The listing builds one solid part. Answer for the finished solid, in the listing's coordinates (mm). Round coordinates to 2 decimals unless told otherwise and drop trailing zeros. Loops run counter-clockwise (first coordinate to the right, second up) from the corner with the lowest first, then second, coordinate; pieces in that order, holes last. Notation, with made-up numbers: (34, 25) - (52, 25) arc R26 cw to (52, 51) - close; hole circle Ø3 at (-26.5, 60). An arc over 180 degrees is marked (long way). One line per item, written item: value.
```python
from build123d import *

# Parameters (mm, degrees)
CYLINDER964_R          = 74
CYLINDER964_DEPTH      = 32
BOX476_W               = 50
BOX476_H               = 6
BOX476_DEPTH           = 26
CUT443_PLACEMENT_ANGLE = 90


with BuildPart() as obj1:
    # Cylinder964 → Cylinder964 (new body)
    with BuildSketch(Plane.XY.offset(50)):
        Circle(CYLINDER964_R)
    extrude(amount=CYLINDER964_DEPTH)


with BuildPart() as cut443:
    # Box476 → Box476 (new body)
    with BuildSketch(Plane(origin=(-112, -24, 56), x_dir=(1, 0, 0), z_dir=(0, 0, 1))):
        with Locations((25, 3)):
            Rectangle(BOX476_W, BOX476_H)
    extrude(amount=BOX476_DEPTH)

    # Cut443: cut obj1
    add(obj1.part, mode=Mode.SUBTRACT)


with BuildPart() as cut443_1:
    # Cut443 placement: moved
    add(cut443.part.rotate(Axis((0, 0, 0), (0, 0, 1)), CUT443_PLACEMENT_ANGLE))


solid = cut443_1.part
```
1) A cutting plane is placed at B-B on x = 21. Give the vertices of the cut face in (y, z), and give its area (3 significant figures).
Final values:
outline: (-112, 56) - (-70.96, 56) - (-70.96, 82) - (-112, 82) - close
area: 1,070 mm2
2) This flat-tipped pin is pushed along its axis until it touches: pin 1 Ø3 at (x, z) = (23, 75.5) entering from +Y. Where does it stop, or does it pass through?
Final values:
pin 1: y = -70
3) A cutting plane is placed at A-A on z = 59.5. Give the vertices of the cut face in (x, y), and give its area (3 significant figures).
Final values:
outline: (18, -112) - (24, -112) - (24, -70) arc R74 cw to (18, -71.78) - close
area: 246 mm2
4) Consider L1, parallel to Y at x = 23, z = 68.25; L2, parallel to Y at x = 20.5, z = 58.75. Determine where each line is inside the solid, lowest interval first.
Final values:
L1: -112 to -70.33
L2: -112 to -71.1
